The listing builds one solid part. Answer for the finished solid, in the listing's coordinates (mm). Face numbers are marked on the shaded views. Coordinates: 2 decimals unless noted, no trailing zeros. Write each loop counter-clockwise with the first axis right and the second up, starting at its lowest first coordinate (ties: lowest second). Pieces come first, ordered by that corner, then holes. Notation, with made-up numbers: M -22,70 L 16,70 A11 ccw 16,88 Z; hole C 45.25,21 d4. An arc over 180 degrees is marked long. Answer as CSV lines item,"result".
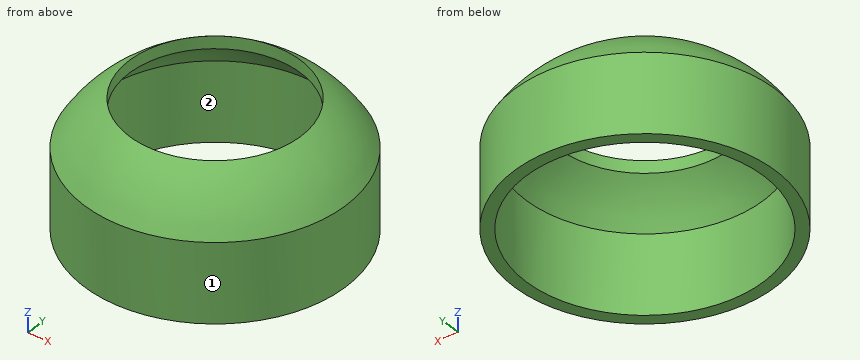
```python
from build123d import *

# Parameters (mm, degrees)
SKETCH_R   = 23.2
SKETCH_R_2 = 21.1
PAD_DEPTH  = 14


with BuildPart() as body001:
    # Sketch001 → Revolution (revolve)
    with BuildSketch(Plane.XZ):
        with BuildLine():
            ThreePointArc((-15.2, 20.252654), (-18.417286, 17.378538), (-21.1, 14))
            Line((-21.1, 14), (-23.2, 14))
            ThreePointArc((-15.2, 22.43212), (-19.657445, 18.650063), (-23.2, 14))
            Line((-15.2, 20.252654), (-15.2, 22.43212))
        make_face()
    revolve(axis=Axis((0, 0, 0), (0, 0, 1)))


with BuildPart() as body:
    # Sketch → Pad (new body)
    with BuildSketch(Plane.XY):
        Circle(SKETCH_R)
        Circle(SKETCH_R_2, mode=Mode.SUBTRACT)
    extrude(amount=PAD_DEPTH)

    # Boolean: union Body001
    add(body001.part)


solid = body.part
```
Q1. Flat-ended cylindrical pins translate along their axes: pin 1 Ø8 at (x, z) = (-15, 12) entering from +Y; pin 2 Ø3 at (x, z) = (14.5, 13) entering from -Y; pin 3 Ø12 at (x, z) = (15.5, 2.5) entering from -Y; pin 4 Ø18 at (x, y) = (0, 0) entering from +Z. Find the tip coordinate at first contact, or state that the pin passes through.
Output:
pin 1,"y = 20.43"
pin 2,"y = -19.22"
pin 3,"y = -21.17"
pin 4,"through"
Q2. The mould has two halves that part along X. Classify the marked faces 1 and 2: pulls with the +X half, pulls with the -X half, needs draft (parallel to the pull), parting line crosses it, or undercut.
Output:
face 1,"parting line crosses it"
face 2,"undercut"
Q3. Find section A-A (z = 6.5). Give the vertices of the cut face in (x, y).
Output:
outline,"C 0,0 d46.4; hole C 0,0 d42.2"
Q4. Straight lines are drawn through the part: line 1 (Y direction, x = 0, z = 8.25); line 2 (X direction, y = -9, z = 9.25). For each, find the intervals that lie inside material, in ascending order.
Output:
line 1,"-23.2 to -21.1, 21.1 to 23.2"
line 2,"-21.38 to -19.08, 19.08 to 21.38"
